```python
from build123d import *

# Parameters (mm, degrees)
SKETCH_1_R           = 22.5
SKETCH_1_R_2         = 5
EXTRUDE_1_DEPTH      = 12
SKETCH_2_R           = 1.5
CUT_EXTRUDE_1_DEPTH  = 5.5
CHAMFER_1_SIZE       = 0.5
SKETCH_3_OUTSIDE_W   = 59.952
SKETCH_3_OUTSIDE_H   = 59.952
SKETCH_3_OUTSIDE_W_2 = 37.8
SKETCH_3_OUTSIDE_H_2 = 50
CUT_EXTRUDE_2_DEPTH  = 9.5
SKETCH_4_R           = 8
SKETCH_4_R_2         = 4
EXTRUDE_2_DEPTH      = 16
SKETCH_5_R           = 2
SKETCH_5_R_2         = 1.65
CUT_EXTRUDE_3_DEPTH  = 16.5


with BuildPart() as part:
    # 草图1 → 凸台-拉伸1 (new body)
    with BuildSketch(Plane.XY):
        Circle(SKETCH_1_R)
        Circle(SKETCH_1_R_2, mode=Mode.SUBTRACT)
    extrude(amount=EXTRUDE_1_DEPTH)

    # 草图2 → 切除-拉伸1 (cut)
    with BuildSketch(Plane.XY.offset(12)):
        with Locations((12.02081528, 12.02081528)):
            Circle(SKETCH_2_R)
        with Locations((12.02081528, -12.02081528)):
            Circle(SKETCH_2_R)
        with Locations((-12.02081528, -12.02081528)):
            Circle(SKETCH_2_R)
        with Locations((-12.02081528, 12.02081528)):
            Circle(SKETCH_2_R)
    extrude(amount=-CUT_EXTRUDE_1_DEPTH, mode=Mode.SUBTRACT)

    # 倒角1
    chamfer_1_edges = [part.edges().sort_by_distance(p)[0] for p in [
        (-22.5, 0, 12),
    ]]
    chamfer(chamfer_1_edges, length=CHAMFER_1_SIZE)

    # 草图3 outside → 切除-拉伸2 (cut)
    with BuildSketch(Plane(origin=(0, 0, 0), x_dir=(-1, 0, 0), z_dir=(0, 0, -1))):
        Rectangle(SKETCH_3_OUTSIDE_W, SKETCH_3_OUTSIDE_H)
        Rectangle(SKETCH_3_OUTSIDE_W_2, SKETCH_3_OUTSIDE_H_2, mode=Mode.SUBTRACT)
    extrude(amount=-CUT_EXTRUDE_2_DEPTH, mode=Mode.SUBTRACT)

    # 草图4 → 凸台-拉伸2 (add)
    with BuildSketch(Plane(origin=(0, 0, 0), x_dir=(-1, 0, 0), z_dir=(0, 0, -1))):
        with Locations(Location((0, 0, 0), (0, 0, 180))):
            Circle(SKETCH_4_R)
        Circle(SKETCH_4_R_2, mode=Mode.SUBTRACT)
    extrude(amount=EXTRUDE_2_DEPTH)

    # 草图5 → 切除-拉伸3 (cut)
    with BuildSketch(Plane(origin=(0, 0, 0), x_dir=(-1, 0, 0), z_dir=(0, 0, -1))):
        with Locations((0, 16)):
            Circle(SKETCH_5_R)
        with Locations((0, -16)):
            Circle(SKETCH_5_R_2)
    extrude(amount=-CUT_EXTRUDE_3_DEPTH, mode=Mode.SUBTRACT)


solid = part.part
```
Here's how the part is built. I have some questions about the finished solid (model axes, mm). A direction names the side the tool comes from. Coordinates: 2 decimals unless noted, no trailing zeros. Order: outer loops, then holes, each group sorted by start corner. A loop starts at its lowest first (then second) coordinate and runs counter-clockwise, first axis right, second up.
1) Imagine slicing it at D-D on x = -0.5. State how many separate pieces and enclosed holes the cut face has, and give its area (3 significant figures).
2) Will these pins go through, and if not, where does the flat tip stop? pin 1 (6 mm diameter, centred on x = -13.5, z = 4.5, fed in from -Y); pin 2 (10 mm diameter, centred on x = 15, z = -5.5, fed in from -Y); pin 3 (3 mm diameter, centred on y = 6, z = 6.5, fed in from +X); pin 4 (7.5 mm diameter, centred on y = 6, z = 5.5, fed in from -X).
3) Imagine slicing it at A-A on z = 1. List the corners of the cut face in (x, y) for me.
4) We'd pull the mould along X, two halves only. Please class faces 1 (the face through (12, -12, 6.5)), 2 (the face through (-5.2, 0.3, 12)), 3 (the face through (18.9, 0, 5)): +X half, -X half, draft (parallel to the pull), parting line (faces both ways), or undercut.
5) I need wall thicknesses on line 1 (Y direction, x = 0, z = 5); line 2 (Z direction, x = 7.5, y = -15); line 3 (X direction, y = -12, z = 3.25). Which ranges of each line are inside material? Lowest first, please.
6) Which directions (+Z, -Z, +X, -X, +Y, -Y) give clear straight access to the entire face, cutting with the end or side of a thin tool? Please do faces 4 (the face through (-1.73, 7.81, -7.89)), 5 (the face through (12, 12, 6.5)), 6 (the face through (-20, 0, 9.5)), 7 (the face through (20, 0, 9.5)).
7) Imagine slicing it at C-C on z = -5.25. List the corners of the cut face in (x, y) for me, and give its area (3 significant figures).
8) Imagine slicing it at B-B on y = 0. List the corners of the cut face in (x, z) for me, and give its area (3 significant figures).
Response values:
1. separate pieces: 4
1. enclosed holes: 0
1. area: 465 mm2
2. pin 1: stops at y = -19.9
2. pin 2: passes through
2. pin 3: stops at x = 18.9
2. pin 4: stops at x = -18.9
3. outline: (-18.9, -12.21) arc R22.5 ccw to (18.9, -12.21) - (18.9, 12.21) arc R22.5 ccw to (-18.9, 12.21) - close; hole circle Ø10 at (0, 0); hole circle Ø4 at (0, 16); hole circle Ø3.3 at (0, -16)
4. face 1: undercut
4. face 2: draft
4. face 3: +X half
5. line 1: y = -22.5 to -17.65, -14.35 to -5, 5 to 14, 18 to 22.5
5. line 2: z = 0 to 12
5. line 3: x = -18.9 to 18.9
6. face 4: -Z
6. face 5: +Z
6. face 6: -Z, -X, +Y, -Y
6. face 7: -Z, +X, +Y, -Y
7. outline: circle Ø16 at (0, 0); hole circle Ø8 at (0, 0)
7. area: 151 mm2
8. outline: (-22.5, 9.5) - (-18.9, 9.5) - (-18.9, 0) - (-8, 0) - (-8, -16) - (-4, -16) - (-4, 0) - (-5, 0) - (-5, 12) - (-22, 12) - (-22.5, 11.5) - close; (4, -16) - (8, -16) - (8, 0) - (18.9, 0) - (18.9, 9.5) - (22.5, 9.5) - (22.5, 11.5) - (22, 12) - (5, 12) - (5, 0) - (4, 0) - close
8. area: 479 mm2
